from build123d import *

# Parameters (mm, degrees)
F1_DEPTH    = 3.175
F2_R        = 5.08
F3_R        = 3.175
F4_DEPTH    = 25.4
F5_T1_DEPTH = 118.410793948
F5_T3_DEPTH = 67.600521864
F5_T5_DEPTH = 118.4005208253
F5_T7_DEPTH = 67.6005208253


# Not quite as in the source:
# - a fillet or chamfer that OpenCascade refuses, or shapes differently, is made with other operations: its cross-section is extruded or revolved along the edge and cut away or added


with BuildPart() as f1:
    # F0 (on Front) → F1 (new body, symmetric)
    with BuildSketch(Plane.XZ):
        Polygon((52.0995333791, 24.9929322481), (-49.5107397437, 24.9929322481), (-49.5107397437, -25.8070677519), (52.0892602563, -25.8070677519), align=None)
    extrude(amount=F1_DEPTH, both=True)

    # F2
    f2_edges = [f1.edges().sort_by_distance(p)[0] for p in [
        (-49.51074, -3.175, -0.407068),
        (1.294397, -3.175, 24.992932),
        (52.094397, -3.175, -0.407068),
        (1.28926, -3.175, -25.807068),
    ]]
    fillet(f2_edges, radius=F2_R)

    # F3 (on face) → F4 (cut)
    with BuildSketch(Plane.XZ.offset(3.175)):
        with Locations((-38.2700785995, 15.264518559)):
            Circle(F3_R)
    extrude(amount=-F4_DEPTH, mode=Mode.SUBTRACT)

    # F5: fillet of radius 5.08 on 4 edges, made by hand

    # F5_s2 → F5_t1 (cut)
    with BuildSketch(Plane.YZ.offset(-57.9110001563)):
        with BuildLine():
            ThreePointArc((1.905, 24.9929322481), (2.8469048812, 23.4288793073), (3.175, 21.6328280831))
            Line((3.175, 21.6328280831), (3.175, 24.9929322481))
            Line((3.175, 24.9929322481), (1.905, 24.9929322481))
        make_face()
    extrude(amount=F5_T1_DEPTH, mode=Mode.SUBTRACT)

    # F5_s4 → F5_t3 (cut)
    with BuildSketch(Plane(origin=(-0.0069155089, 0, -34.196793092), x_dir=(0, 1, 0), z_dir=(0.0002022268, 0, 0.9999999796))):
        with BuildLine():
            ThreePointArc((3.175, -48.7343739074), (2.8469048812, -50.5304251316), (1.905, -52.0944780725))
            Line((1.905, -52.0944780725), (3.175, -52.0944780725))
            Line((3.175, -52.0944780725), (3.175, -48.7343739074))
        make_face()
    extrude(amount=F5_T3_DEPTH, mode=Mode.SUBTRACT)

    # F5_s6 → F5_t5 (cut)
    with BuildSketch(Plane.YZ.offset(-57.9110001563)):
        with BuildLine():
            ThreePointArc((3.175, -22.4469635868), (2.8469048812, -24.243014811), (1.905, -25.8070677519))
            Line((1.905, -25.8070677519), (3.175, -25.8070677519))
            Line((3.175, -25.8070677519), (3.175, -22.4469635868))
        make_face()
    extrude(amount=F5_T5_DEPTH, mode=Mode.SUBTRACT)

    # F5_s8 → F5_t7 (cut)
    with BuildSketch(Plane.XY.offset(-34.2073281645)):
        with BuildLine():
            ThreePointArc((-49.5107397437, 1.905), (-47.9466868029, 2.8469048812), (-46.1506355787, 3.175))
            Line((-46.1506355787, 3.175), (-49.5107397437, 3.175))
            Line((-49.5107397437, 3.175), (-49.5107397437, 1.905))
        make_face()
    extrude(amount=F5_T7_DEPTH, mode=Mode.SUBTRACT)


solid = f1.part
Verification items for the finished model (mm, model axes). Coordinates: 2 decimals unless noted, no trailing zeros. Loops run counter-clockwise (first coordinate to the right, second up) from the corner with the lowest first, then second, coordinate; pieces in that order, holes last. Notation, with made-up numbers: M -31.5,43.5 L 27.5,43.5 A18 ccw 27.5,49.5 Z; hole C -5,69 d4. An arc over 180 degrees is marked long. One line per item, written item: value.
1. Mould release check, pull along Z, two halves, no side actions. Record for faces 1 (the cylindrical face through (0.578, 2.856, -24.219)), 2 (the cylindrical face through (-35.337, -0.044, 14.048)), 3 (the cylindrical face through (0.58, 2.84, 23.45)), 4 (the cylindrical face through (-47.98, -1.73, -0.76)): pulls with the +Z half, pulls with the -Z half, needs draft (parallel to the pull), parting line crosses it, or undercut.
Answers follow:
face 1: pulls with the -Z half
face 2: undercut
face 3: pulls with the +Z half
face 4: needs draft
2. Material ranges on line 1 along X through (y, z) = (1.5, -4.5); line 2 along Z through (x, y) = (19, 1.75); line 3 along Z through (x, y) = (-39, -2), recorded low to high. Write a range as from..to.
Answers follow:
line 1: -49.49..52.08
line 2: -25.8..24.99
line 3: -23.98..12.17, 18.35..23.16
3. Section check B-B on x = 33. Record the cut outline in (y, z) (3 decimals).
Answers follow:
outline: M -3.175,-20.727 A5.08 ccw 1.905,-25.807 A5.08 ccw 3.175,-22.447 L 3.175,21.633 A5.08 ccw 1.905,24.993 A5.08 ccw -3.175,19.913 Z
4. Gauge pin test, flat ends, axial feed: P1, Ø3, axis at y = -1.5, z = -10.5, coming from the -X side; P2, Ø1, axis at y = 0, z = -18, coming from the +X side. Record the tip position at first contact, or that the pin passes through.
Answers follow:
P1: x = -49.14
P2: x = 51.89
5. Section check A-A on y = -0.25. Record the cut outline in (x, z) (3 decimals), plus the area to 3 significant figures.
Answers follow:
outline: M -49.031,-25.327 L 51.61,-25.327 L 51.62,24.513 L -49.031,24.513 Z; hole C -38.27,15.265 d6.35
area: 4,980 mm^2
